Check sheet for the modelled part. Datum: model origin and axes. Units: mm. A direction names the side the tool comes from. Coordinates: 2 decimals unless noted, no trailing zeros. Loops run counter-clockwise (first coordinate to the right, second up) from the corner with the lowest first, then second, coordinate; pieces in that order, holes last.
Autodesk Inventor part; units mm, degrees
ref_plane "YZ Plane" through (0, 0, 0) normal (1, 0, 0) x (0, 1, 0)
ref_plane "XZ Plane" through (0, 0, 0) normal (0, 1, 0) x (-1, 0, 0)
ref_plane "XY Plane" through (0, 0, 0) normal (0, 0, 1) x (1, 0, 0)
sketch "本体面" plane through (0, 0, 0) normal (0, 0, 1) x (1, 0, 0)
  line L0 (-11.6, 17) -> (11.6, 17)
  line L1 (11.6, 17) -> (11.6, 0)
  line L2 (11.6, 0) -> (-11.6, 0)
  line L3 (-11.6, 0) -> (-11.6, 17)
  point P0 (0, 0)
  point P1 (0, 0)
  dimension "d0" = 23.2
  dimension "d1" = 17
extrude "本体" add sketch "本体面" along normal blind 32
sketch "空洞面" plane through (0, 0, 32) normal (0, 0, 1) x (1, 0, 0)
  line L0 (-9.3, 11) -> (9.3, 11)
  line L1 (9.3, 11) -> (9.3, 3)
  line L2 (7.3, 1) -> (-7.3, 1)
  line L3 (-9.3, 3) -> (-9.3, 11)
  line L4 (11.6, 17) -> (-11.6, 17)
  arc A0 (-9.3, 3) -> (-7.3, 1) centre (-7.3, 3) ccw
  arc A1 (7.3, 1) -> (9.3, 3) centre (7.3, 3) ccw
  line L5 (-11.6, 0) -> (11.6, 0)
  point P0 (0, 0)
  point P1 (9.3, 1)
  point P2 (-9.3, 1)
  point P3 (0, 11)
  dimension "d4" = 18.6
  dimension "d6" = 2
  dimension "d31" = 1
  dimension "d32" = 10
extrude "空洞" cut sketch "空洞面" against normal blind 32
sketch "左溝面" plane through (0, 0, 32) normal (0, 0, 1) x (1, 0, 0)
  line L0 (-10.6, 10.2) -> (-9.3, 10.2)
  line L1 (-9.3, 10.2) -> (-9.3, 8.2)
  line L2 (-9.3, 8.2) -> (-10.6, 8.2)
  line L3 (-10.6, 8.2) -> (-10.6, 10.2)
  line L4 (11.6, 17) -> (-11.6, 17) construction
  line L5 (-11.6, 17) -> (-11.6, 0) construction
  line L6 (-9.3, 3) -> (-9.3, 11) construction
  line L7 (-9.3, 11) -> (9.3, 11) construction
  point P0 (0, 0)
  point P1 (-9.3, 28)
  dimension "d10" = 2
  dimension "d28" = 1
  dimension "d33" = 0.8
extrude "左溝" cut sketch "左溝面" against normal blind 31
sketch "右溝面" plane through (0, 0, 32) normal (0, 0, 1) x (1, 0, 0)
  line L0 (9.3, 10.2) -> (10.6, 10.2)
  line L1 (10.6, 10.2) -> (10.6, 8.2)
  line L2 (10.6, 8.2) -> (9.3, 8.2)
  line L3 (9.3, 8.2) -> (9.3, 10.2)
  line L4 (11.6, 0) -> (11.6, 17) construction
  line L5 (9.3, 11) -> (9.3, 3) construction
  line L6 (-9.3, 11) -> (9.3, 11) construction
  point P0 (0, 0)
  dimension "d22" = 2
  dimension "d30" = 1
  dimension "d34" = 0.8
extrude "右溝" cut sketch "右溝面" against normal blind 31
sketch "穴面" plane through (0, 0, 0) normal (0, 0, -1) x (-1, 0, 0)
  line L0 (-7.3, 15) -> (7.3, 15)
  line L1 (9.3, 13) -> (9.3, 4)
  line L2 (7.3, 2) -> (-7.3, 2)
  line L3 (-9.3, 4) -> (-9.3, 13)
  line L4 (11.6, 17) -> (-11.6, 17) construction
  line L5 (-11.6, 0) -> (11.6, 0) construction
  arc A0 (-7.3, 15) -> (-9.3, 13) centre (-7.3, 13) ccw
  arc A1 (9.3, 13) -> (7.3, 15) centre (7.3, 13) ccw
  arc A2 (-9.3, 4) -> (-7.3, 2) centre (-7.3, 4) ccw
  arc A3 (7.3, 2) -> (9.3, 4) centre (7.3, 4) ccw
  line L6 (9.3, 11) -> (9.3, 3)
  line L7 (-9.3, 3) -> (-9.3, 11)
  point P0 (0, 0)
  dimension "d41" = 2
  dimension "d44" = 2
  dimension "d45" = 2
sketch "スケッチ11" plane through (0, 0, 32) normal (0, 0, 1) x (1, 0, 0)
  line L0 (-11.6, 17) -> (11.6, 17)
  line L1 (11.6, 17) -> (11.6, 0)
  line L2 (-11.6, 17) -> (11.6, 17)
  line L3 (11.6, 17) -> (11.6, 10.9937)
  line L4 (11.6, 10.9937) -> (-11.6, 10.9937)
  line L5 (-11.6, 10.9937) -> (-11.6, 17)
  point P0 (0, 0)
extrude "押し出し9" cut sketch "スケッチ11" along normal through all both and the other way through all
sketch "スケッチ12" plane through (-7.3, 1, 32) normal (0, 1, 0) x (1, 0, 0)
  line L0 (14.6, 0) -> (0, 0)
  line L1 (0, 0) -> (0, 32)
  line L2 (0, 0) -> (-2, 0)
  line L3 (14.6, 0) -> (14.6, 32)
  circle A0 centre (7.3, 16) radius 1.5
  point P0 (7.3, 32)
  dimension "d65" = 3
extrude "押し出し10" cut sketch "スケッチ12" against normal through all
properties part number "HB5_holder"
1) Section check B-B on y = 3.5. Enter the section's corners in (x, z).
Answer sheet:
outline: (-11.6, 0) - (-9.3, 0) - (-9.3, 32) - (-11.6, 32) - close; (9.3, 0) - (11.6, 0) - (11.6, 32) - (9.3, 32) - close
2) Section check A-A on z = 16. Enter the section's corners in (x, y).
Answer sheet:
outline: (-11.6, 0) - (-1.5, 0) - (-1.5, 1) - (-7.3, 1) arc R2 cw to (-9.3, 3) - (-9.3, 8.2) - (-10.6, 8.2) - (-10.6, 10.2) - (-9.3, 10.2) - (-9.3, 10.99) - (-11.6, 10.99) - close; (1.5, 0) - (11.6, 0) - (11.6, 10.99) - (9.3, 10.99) - (9.3, 10.2) - (10.6, 10.2) - (10.6, 8.2) - (9.3, 8.2) - (9.3, 3) arc R2 cw to (7.3, 1) - (1.5, 1) - close
3) Set-up check for faces 4 (the flat face through (2, 1, 16)), 5 (the flat face through (-0.1, 0.2, 0)), 6 (the flat face through (10.6, 9, 17)): record each of +Z, -Z, +X, -X, +Y, -Y from which the full face is reachable in a straight line by a thin tool's end or side.
Answer sheet:
face 4: +Z, -Z, +Y
face 5: -Z, +X, -X, +Y, -Y
face 6: +Z
4) Scan lines: line 1 (X direction, y = 3, z = 2.5); line 2 (X direction, y = 0.45, z = 16); line 3 (Z direction, x = 0, y = 0.35). Record each from-to range of solid material in increasing order.
Answer sheet:
line 1: x = -11.6 to -9.3, 9.3 to 11.6
line 2: x = -11.6 to -1.5, 1.5 to 11.6
line 3: z = 0 to 14.5, 17.5 to 32
5) Section check D-D on z = 3.5. Enter the section's corners in (x, y), plus the area to 3 significant figures.
Answer sheet:
outline: (-11.6, 0) - (11.6, 0) - (11.6, 10.99) - (9.3, 10.99) - (9.3, 10.2) - (10.6, 10.2) - (10.6, 8.2) - (9.3, 8.2) - (9.3, 3) arc R2 cw to (7.3, 1) - (-7.3, 1) arc R2 cw to (-9.3, 3) - (-9.3, 8.2) - (-10.6, 8.2) - (-10.6, 10.2) - (-9.3, 10.2) - (-9.3, 10.99) - (-11.6, 10.99) - close
area: 65.7 mm2
6) Depth check by flat-ended pin: pin 1 (0.6 mm diameter, centred on x = -9.5, z = 11, fed in from -Y); pin 2 (4.5 mm diameter, centred on x = -3, z = 12, fed in from +Y); pin 3 (0.6 mm diameter, centred on x = -10, y = 9.5, fed in from +Z). Enter the tip coordinate at first touch or a pass-through.
Answer sheet:
pin 1: stops at y = 0
pin 2: stops at y = 1
pin 3: stops at z = 1
7) Section check C-C on x = 0. Enter the section's corners in (y, z), plus the area to 3 significant figures.
Answer sheet:
outline: (0, 0) - (1, 0) - (1, 14.5) - (0, 14.5) - close; (0, 17.5) - (1, 17.5) - (1, 32) - (0, 32) - close
area: 29.0 mm2
8) Mould release check, pull along X, two halves, no side actions. Record for faces 1 (the flat face through (-11.6, 5, 16)), 2 (the flat face through (3, 0, 16)), 3 (the flat face through (10, 8.2, 17)): +X half, -X half, draft (parallel to the pull), parting line (faces both ways), or undercut.
Answer sheet:
face 1: -X half
face 2: draft
face 3: undercut
